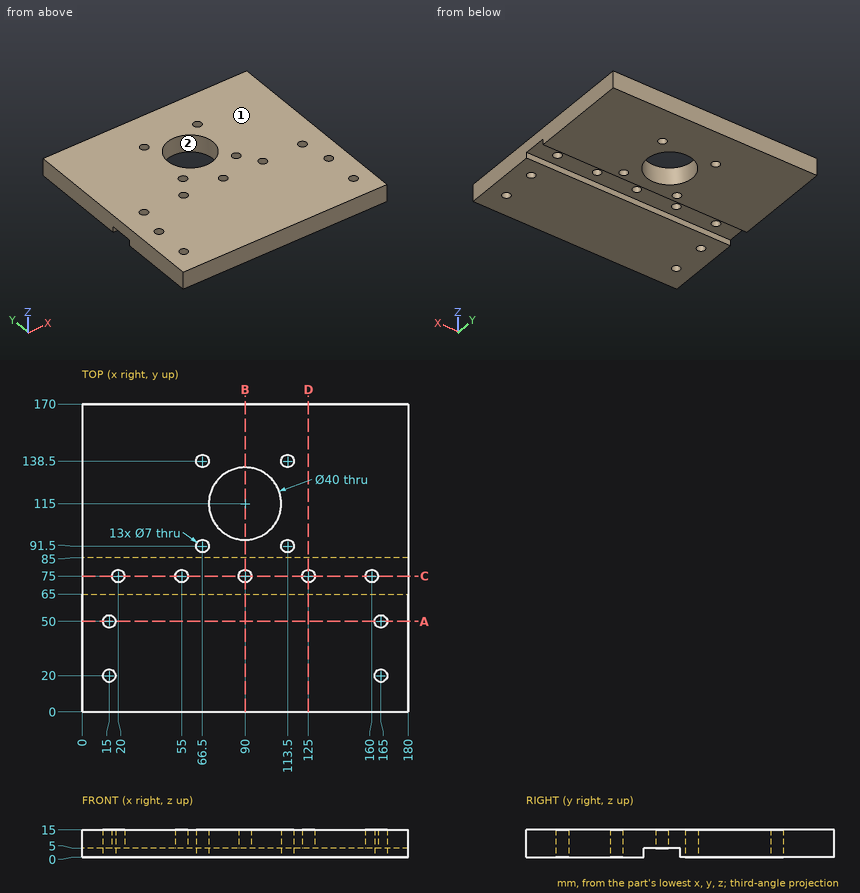
Here's the drawing with two shaded views (mm, measured from the low corner). I have some questions. Coordinates: 2 decimals unless noted, no trailing zeros. Loops run counter-clockwise (first coordinate to the right, second up) from the corner with the lowest first, then second, coordinate; pieces in that order, holes last. Notation, with made-up numbers: (17.5, 39.25) -> (63.5, 39.25) arc R22 ccw to (63.5, 57.25) -> close; hole circle Ø8 at (-18.5, 27). An arc over 180 degrees is marked (long way). Answer in a Markdown table with one row per item.
(1) If I drill on probe 1 along Y at (x, z) = (90, 9.75); probe 2 along X at (y, z) = (138.5, 12); probe 3 along Y at (x, z) = (165, 3.5), over which ranges is the centre line in solid material (lowest first)?
Results found:
| item | result |
|---|---|
| probe 1 | y = 0 to 71.5, 78.5 to 95, 135 to 170 |
| probe 2 | x = 0 to 63, 70 to 110, 117 to 180 |
| probe 3 | y = 0 to 16.5, 23.5 to 46.5, 53.5 to 65, 85 to 170 |
(2) Imagine slicing it at A-A (y = 50). List the corners of the cut face in (x, z) for me, plus the area to 3 significant figures.
Results found:
| item | result |
|---|---|
| outline | (0, 0) -> (11.5, 0) -> (11.5, 15) -> (0, 15) -> close; (18.5, 0) -> (161.5, 0) -> (161.5, 15) -> (18.5, 15) -> close; (168.5, 0) -> (180, 0) -> (180, 15) -> (168.5, 15) -> close |
| area | 2,490 mm^2 |
(3) Imagine slicing it at D-D (x = 125). List the corners of the cut face in (y, z) for me, plus the area to 3 significant figures.
Results found:
| item | result |
|---|---|
| outline | (0, 0) -> (65, 0) -> (65, 5) -> (71.5, 5) -> (71.5, 15) -> (0, 15) -> close; (78.5, 5) -> (85, 5) -> (85, 0) -> (170, 0) -> (170, 15) -> (78.5, 15) -> close |
| area | 2,380 mm^2 |
(4) Imagine slicing it at B-B (x = 90). List the corners of the cut face in (y, z) for me.
Results found:
| item | result |
|---|---|
| outline | (0, 0) -> (65, 0) -> (65, 5) -> (71.5, 5) -> (71.5, 15) -> (0, 15) -> close; (78.5, 5) -> (85, 5) -> (85, 0) -> (95, 0) -> (95, 15) -> (78.5, 15) -> close; (135, 0) -> (170, 0) -> (170, 15) -> (135, 15) -> close |
(5) Thinking about a two-plate mould opening in Y: for the marked faces 1 and 2, which applies, released by +Y, released by -Y, zero draft, split by the parting line, or undercut?
Results found:
| item | result |
|---|---|
| face 1 | zero draft |
| face 2 | undercut |
(6) Imagine slicing it at C-C (y = 75). List the corners of the cut face in (x, z) for me.
Results found:
| item | result |
|---|---|
| outline | (0, 5) -> (16.5, 5) -> (16.5, 15) -> (0, 15) -> close; (23.5, 5) -> (51.5, 5) -> (51.5, 15) -> (23.5, 15) -> close; (58.5, 5) -> (86.5, 5) -> (86.5, 15) -> (58.5, 15) -> close; (93.5, 5) -> (121.5, 5) -> (121.5, 15) -> (93.5, 15) -> close; (128.5, 5) -> (156.5, 5) -> (156.5, 15) -> (128.5, 15) -> close; (163.5, 5) -> (180, 5) -> (180, 15) -> (163.5, 15) -> close |
(7) Will these pins go through, and if not, where does the flat tip stop? pin 1 Ø5.5 at (x, y) = (90, 75) entering from -Z; pin 2 Ø8 at (x, y) = (20, 75) entering from -Z.
Results found:
| item | result |
|---|---|
| pin 1 | passes through |
| pin 2 | stops at z = 5 |
